Autodesk Inventor part; units mm, degrees
ref_plane "Work Plane1" through (0, 0, 5) normal (0, 0, 1) x (1, 0, 0)
ref_plane "YZ Plane" through (0, 0, 0) normal (1, 0, 0) x (0, 1, 0)
ref_plane "XZ Plane" through (0, 0, 0) normal (0, 1, 0) x (-1, 0, 0)
sketch "Sketch1" plane through (0, 0, 0) normal (0, 0, 1) x (1, 0, 0)
  circle A0 centre (0, 0) radius 4
  circle A1 centre (0, 0) radius 5
  line L0 (-90, -6) -> (90, -6)
  line L1 (90, -6) -> (90, 6)
  line L2 (90, 6) -> (-90, 6)
  line L3 (-90, 6) -> (-90, -6)
  line L4 (-90, -6) -> (90, 6) construction
  line L5 (90, -6) -> (-90, 6) construction
  point P0 (0, -5)
  point P1 (0, 5)
  point P2 (0, 0)
  point P3 (0, 0)
  dimension "d11" = 180
  dimension "d14" = 12
ref_plane "Work Plane1" through (0, 0, 5) normal (0, 0, 1) x (1, 0, 0)
extrude "Extrusion3" add sketch "Sketch1" along normal mid plane 10 contours A0 | A1 | L3 L2 L1 L0
extrude "Extrusion4" cut sketch "Sketch1" along normal mid plane 10 contours A0
fillet "Fillet3" radius 6 4 edges at (-90, -6, 0) (-90, 6, 0) (90, 6, 0) (90, -6, 0)
sketch "Sketch4" plane through (0, 0, 5) normal (0, 0, 1) x (1, 0, 0)
  circle A0 centre (0, 0) radius 4
  line L0 (0, 0) -> (-80, 0)
  circle A1 centre (-80, 0) radius 4
  circle A2 centre (-80, 0) radius 6
  line L1 (-84, 6) -> (84, 6)
  point P0 (0, 0)
  dimension "d22" = 80
  dimension "d23" = 8
extrude "Extrusion6" cut sketch "Sketch4" against normal blind 10 contours A1
mirror "Mirror2" about plane through (0, 0, 0) normal (1, 0, 0) of "Extrusion6"
properties part number "Lever"
Part model, mm, in its own coordinate system. Give positions to 0.01 mm unless a question says otherwise; leave off trailing zeros. Order: outer loops, then holes, each group sorted by start corner. A loop starts at its lowest first (then second) coordinate and runs counter-clockwise, first axis right, second up. Notation, with made-up numbers: (-7.75, 79) - (30.25, 79) arc R15 ccw to (30.25, 91) - close; hole circle Ø7 at (10, 12.5). An arc over 180 degrees is marked (long way). Use a Markdown table: item, result.
1) Two-plate mould, pull along X, no slides. Class faces 1 (the cylindrical face through (-84, 0, 0)), 2 (the flat face through (-1.3, 4.1, -5)), 3 (the cylindrical face through (-88.289, -4.196, 0.07)): +X half, -X half, draft (parallel to the pull), parting line (faces both ways), or undercut.
Checked values:
| item | result |
|---|---|
| face 1 | undercut |
| face 2 | draft |
| face 3 | -X half |
2) Saw through at C-C on y = -2.5. List the corners of the cut face in (x, z).
Checked values:
| item | result |
|---|---|
| outline | (-89.45, -5) - (-83.12, -5) - (-83.12, 5) - (-89.45, 5) - close; (-76.88, -5) - (-3.12, -5) - (-3.12, 5) - (-76.88, 5) - close; (3.12, -5) - (76.88, -5) - (76.88, 5) - (3.12, 5) - close; (83.12, -5) - (89.45, -5) - (89.45, 5) - (83.12, 5) - close |
3) Probe L1, parallel to X at y = 0.25, z = 1.5; L2, parallel to Y at x = 80, z = 0.5; L3, parallel to X at y = -1, z = -1.5. List the from-to ranges inside material, lowest first. Write a range as from..to.
Checked values:
| item | result |
|---|---|
| L1 | -89.99..-83.99, -76.01..-3.99, 3.99..76.01, 83.99..89.99 |
| L2 | -6..-4, 4..6 |
| L3 | -89.92..-83.87, -76.13..-3.87, 3.87..76.13, 83.87..89.92 |
4) Saw through at B-B on z = -1.75. Count the separate pieces of the cut face and the enclosed holes in it, plus the area to 3 significant figures.
Checked values:
| item | result |
|---|---|
| separate pieces | 1 |
| enclosed holes | 3 |
| area | 1,980 mm² |
5) Saw through at A-A on x = 80. List the corners of the cut face in (y, z).
Checked values:
| item | result |
|---|---|
| outline | (-6, -5) - (-4, -5) - (-4, 5) - (-6, 5) - close; (4, -5) - (6, -5) - (6, 5) - (4, 5) - close |
6) Flat gauge pins, fed straight in: P1, Ø5, axis at y = -0.5, z = -2, coming from the -X side; P2, Ø1, axis at y = -3.5, z = 4, coming from the -X side. Where does each tip first touch, or does it go through?
Checked values:
| item | result |
|---|---|
| P1 | x = -90 |
| P2 | x = -89.2 |
